```python
from build123d import *

# Parameters (mm, degrees)
F1_DEPTH = 4
F2_W     = 54
F2_H     = 18
F3_DEPTH = 3
F4_R     = 3.99999


# Not quite as in the source:
# - a fillet or chamfer is up to 0.001 mm smaller than in the source, because OpenCascade refuses the exact size


with BuildPart() as f1:
    # F0 (on Front) → F1 (new body, symmetric)
    with BuildSketch(Plane.XZ):
        Polygon((-49, 0), (5, 0), (5, 3), (0, 3), (0, 8), (-44, 15.1), (-44, 3), (-49, 3), align=None)
    extrude(amount=F1_DEPTH, both=True)

    # F2 (on face) → F3 (join, through all)
    with BuildSketch(Plane(origin=(0, 0, 0), x_dir=(1, 0, 0), z_dir=(0, 0, -1))):
        with Locations((-22, 0)):
            Rectangle(F2_W, F2_H)
    extrude(amount=-F3_DEPTH)

    # F4 (radius 4 in the source; OpenCascade refuses exactly that, so slightly less here)
    f4_edges = [f1.edges().sort_by_distance(p)[0] for p in [
        (0, -4, 5.5),
        (0, 4, 5.5),
        (-44, 4, 9.05),
        (-44, -4, 9.05),
        (-49, -9, 1.5),
        (-49, 9, 1.5),
        (5, 9, 1.5),
        (5, -9, 1.5),
    ]]
    fillet(f4_edges, radius=F4_R)


solid = f1.part
```
Design review of the part built by this model. Coordinates are the model's own, in mm. A direction names the side the tool comes from. Coordinates: 2 decimals unless noted, no trailing zeros. Order: outer loops, then holes, each group sorted by start corner. A loop starts at its lowest first (then second) coordinate and runs counter-clockwise, first axis right, second up.
1) For faces 4 (the cylindrical face through (-42.859, 2.797, 8.965)), 5 (the cylindrical face through (-42.797, -2.859, 8.965)), 6 (the flat face through (-22, 4, 8)), 7 (the cylindrical face through (-1.141, -2.797, 5.862)), list the 3-axis set-ups (+Z, -Z, +X, -X, +Y, -Y) from which the entire face can be reached by the end or side of a thin tool; tool diameter is ignored.
2) Clearance check with flat-ended pins moving along their axes: pin 1 (4 mm diameter, centred on x = -15, y = -0.5, fed in from +Z); pin 2 (1 mm diameter, centred on x = -27.5, y = -2, fed in from +Z); pin 3 (4 mm diameter, centred on y = -3.5, z = 9.5, fed in from +X). State where each tip first meets the part, or that it passes through.
3) Wall thickness on line 1 along Y through (x, z) = (-32, 4.25); line 2 along Z through (x, y) = (-35, -6.75); line 3 along Y through (x, z) = (-41, 13): over which ranges is each line inside the solid? List them lowest first.
4) Take a section at D-D, the plane y = -8. Give the boundary of the cut face in (x, z).
5) Mouldability with a two-part tool opening along Z and no side actions: class faces 1 (the flat face through (-21.7, -0.1, 11.5)), 2 (the cylindrical face through (-1.141, 2.797, 5.862)), 3 (the flat face through (-22, 0, 0)) as +Z half, -Z half, draft (parallel to the pull), parting line (faces both ways), or undercut.
6) Take a section at B-B, the plane y = 1.5. Give the boundary of the cut face in (x, z).
Returned:
1. face 4: +Z, -X, +Y
1. face 5: +Z, -X, -Y
1. face 6: +Z, +X, -X, +Y
1. face 7: +Z, +X, -Y
2. pin 1: stops at z = 10.74
2. pin 2: stops at z = 12.52
2. pin 3: stops at x = -0.58
3. line 1: y = -4 to 4
3. line 2: z = 0 to 3
3. line 3: y = -3.87 to 3.87
4. outline: (-47.65, 0) - (3.65, 0) - (3.65, 3) - (-47.65, 3) - close
5. face 1: +Z half
5. face 2: draft
5. face 3: -Z half
6. outline: (-49, 0) - (5, 0) - (5, 3) - (-0.29, 3) - (-0.29, 8.05) - (-43.71, 15.05) - (-43.71, 3) - (-49, 3) - close
